Check sheet for the modelled part. Datum: model origin and axes. Units: mm. Face numbers are marked on the shaded views. A direction names the side the tool comes from. Round coordinates to 2 decimals unless told otherwise and drop trailing zeros. Write each loop counter-clockwise with the first axis right and the second up, starting at its lowest first coordinate (ties: lowest second). Pieces come first, ordered by that corner, then holes.
Item 1: Cross-section at A-A on y = 42. Enter the section's corners in (x, z), plus the area to 3 significant figures.
Item 2: Cross-section at D-D on x = 3. Enter the section's corners in (y, z).
Item 3: Material ranges on line 1 (Y direction, x = 7.25, z = 1.65); line 2 (Y direction, x = 31.75, z = 2.6); line 3 (X direction, y = 21.5, z = 6.25), recorded low to high.
Item 4: Cross-section at B-B on x = 15. Enter the section's corners in (y, z).
Item 5: Go/stop test with flat-tipped pins: pin 1 Ø3 at (x, y) = (31.75, 7.25) entering from -Z; pin 2 Ø6 at (y, z) = (26.5, -2) entering from -X; pin 3 Ø1 at (y, z) = (20, -1.5) entering from -X. Record where each tip stops, or that it passes through.
Item 6: Tool access check on the marked faces 1, 2 and 3. Record the directions out of +Z, -Z, +X, -X, +Y, -Y that give a thin tool (end or side, any length) a straight path to the whole face; none if there is none.
Item 7: Release check for a two-part mould opening along Y. For the marked faces 4, 5 and 6 record: +Y half, -Y half, draft (parallel to the pull), parting line (faces both ways), or undercut.
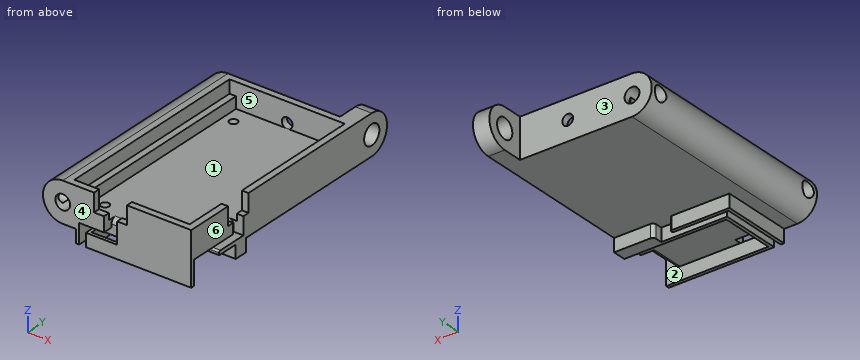
from build123d import *

# Parameters (mm, degrees)
SKETCH1_W                = 39
SKETCH1_H                = 65
BASE_DEPTH               = 4.5
SKETCH2_W                = 4
SKETCH2_H                = 57
WALLS_DEPTH              = 7.5
SKETCH3_W                = 10
SKETCH3_H                = 7.5
PWR_CONNECTOR_HOLE_DEPTH = 4
SKETCH4_W                = 7.5
SKETCH4_H                = 8
GPS_CONNECTOR_HOLE_DEPTH = 4
SKETCH5_R                = 1.25
MOUNTING_HOLES_DEPTH     = 4
GPS_MOUNT_DEPTH          = 4
SKETCH11_W               = 17
SKETCH11_H               = 1
SKETCH11_W_2             = 12
SKETCH11_H_2             = 3
PWR_CABLE_HOLDER1_DEPTH  = 4
SKETCH12_W               = 4
SKETCH12_H               = 2.5
PWR_CABLE_HOLDER2_DEPTH  = 3
PWR_FILLET_R             = 1.5
PWR_FILLET2_R            = 1
PWR_FILLET3_R            = 0.5
GPS_CABLE_HOLDER_DEPTH   = 3
GPS_START                = 1
GPS_FILLET_DEPTH         = 10
GPS_START_2              = 16.5
GPS_FILLET_2_DEPTH       = 4
GPS_START_3              = 9.15727
GPS_FILLET_3_DEPTH       = 8.34273
GPS_FILLET2_R            = 0.5
SKETCH15_R               = 6
BALLON_MOUNT_DEPTH       = 65
SKETCH16_R               = 2.25
BALLOON_MOUNT_HOLE_DEPTH = 65
SKETCH21_R               = 2.25
SAFETY_MOUNT_DEPTH       = 4.5
SKETCH22_W               = 35
SKETCH22_H               = 61
LID_HOLE_DEPTH           = 7.5
SKETCH25_W               = 3.5
SKETCH25_H               = 61
CORRECTION_DEPTH         = 2
SKETCH28_W               = 2
SKETCH28_H               = 2
SKETCH28_W_2             = 3
SMALL_WALLS_DEPTH        = 2
ANTENNA_MOUNTING_DEPTH   = 5
SKETCH30_R               = 3
ANTENNA_HOLE_DEPTH       = 5
SKETCH31_R               = 1.65
CABLE_HOLE_DEPTH         = 2


with BuildPart() as part:
    # Sketch1 → Base (new body)
    with BuildSketch(Plane.XY):
        with Locations((19.5, 32.5)):
            Rectangle(SKETCH1_W, SKETCH1_H)
    extrude(amount=BASE_DEPTH)

    # Sketch2 → Walls (add)
    with BuildSketch(Plane.XY.offset(4.5)):
        Polygon((39, 61), (39, 65), (0, 65), (0, 61), (4, 61), (35, 61), align=None)
        with Locations((37, 32.5)):
            Rectangle(SKETCH2_W, SKETCH2_H)
        Polygon((4, 61), (0, 61), (0, 0), (4, 0), (4, 4), align=None)
        Polygon((39, 0), (39, 4), (35, 4), (4, 4), (4, 0), align=None)
    extrude(amount=WALLS_DEPTH)

    # Sketch3 → PWR connector hole (cut)
    with BuildSketch(Plane(origin=(0, 4, 0), x_dir=(1, 0, 0), z_dir=(0, 1, 0))):
        with Locations((14.5, -8.25)):
            Rectangle(SKETCH3_W, SKETCH3_H)
    extrude(amount=-PWR_CONNECTOR_HOLE_DEPTH, mode=Mode.SUBTRACT)

    # Sketch4 → GPS connector hole (cut)
    with BuildSketch(Plane.ZY.offset(-35)):
        with Locations((8.25, 18.5)):
            Rectangle(SKETCH4_W, SKETCH4_H)
    extrude(amount=-GPS_CONNECTOR_HOLE_DEPTH, mode=Mode.SUBTRACT)

    # Sketch5 → Mounting holes (cut)
    with BuildSketch(Plane.XY.offset(4.5)):
        with Locations((7.25, 7.25)):
            Circle(SKETCH5_R)
        with Locations(Location((31.75, 7.25, 0), (0, 0, 180))):
            Circle(SKETCH5_R)
        with Locations(Location((7.25, 57.75, 0), (0, 0, 180))):
            Circle(SKETCH5_R)
        with Locations((31.75, 57.75)):
            Circle(SKETCH5_R)
    extrude(amount=-MOUNTING_HOLES_DEPTH, mode=Mode.SUBTRACT)

    # Sketch7 → GPS mount (add)
    with BuildSketch(Plane(origin=(0, 0, 0), x_dir=(-1, 0, 0), z_dir=(0, 0, -1))):
        Polygon((-39, 1), (-39, 0), (-7, 0), (-7, 18.5), (-39, 18.5), (-39, 17.5), (-8, 17.5), (-8, 1), align=None)
    extrude(amount=GPS_MOUNT_DEPTH)

    # Sketch11 → PWR cable holder1 (add)
    with BuildSketch(Plane(origin=(0, 0, 0), x_dir=(-1, 0, 0), z_dir=(0, 0, -1))):
        Polygon((-5, 0), (-4, 0), (-4, 21.5), (-5, 21.5), (-5, 20.5), align=None)
        with Locations((-13.5, 21)):
            Rectangle(SKETCH11_W, SKETCH11_H)
        with Locations((-33, 20)):
            Rectangle(SKETCH11_W_2, SKETCH11_H_2)
    extrude(amount=PWR_CABLE_HOLDER1_DEPTH)

    # Sketch12 → PWR cable holder2 (cut)
    with BuildSketch(Plane.XZ):
        Polygon((5, 2), (5, 0), (7, 0), (16.5, 0), (16.5, 2), (12.5, 2), align=None)
        with Locations((14.5, 3.25)):
            Rectangle(SKETCH12_W, SKETCH12_H)
    extrude(amount=-PWR_CABLE_HOLDER2_DEPTH, mode=Mode.SUBTRACT)

    # PWR fillet
    pwr_fillet_edges = [part.edges().sort_by_distance(p)[0] for p in [
        (6, 3, 0),
        (14.5, 3, 4.5),
    ]]
    fillet(pwr_fillet_edges, radius=PWR_FILLET_R)

    # PWR fillet2
    pwr_fillet2_edges = [part.edges().sort_by_distance(p)[0] for p in [
        (27, 21.5, -2),
    ]]
    fillet(pwr_fillet2_edges, radius=PWR_FILLET2_R)

    # PWR fillet3
    pwr_fillet3_edges = [part.edges().sort_by_distance(p)[0] for p in [
        (22, 21.5, -2),
        (22, 20.5, -2),
    ]]
    fillet(pwr_fillet3_edges, radius=PWR_FILLET3_R - 0.0001)  # a hair under: the kernel refuses the full size

    # Sketch13 → GPS cable holder (cut)
    with BuildSketch(Plane(origin=(39, 0, 0), x_dir=(0, 0, -1), z_dir=(1, 0, 0))):
        Polygon((-1.156586719, 11), (-2.326586719, 11), (-2.326586719, 1), (0, 1), (0, 11), align=None)
        Polygon((-2.326586719, 11), (-2.326586719, 16.5), (-3.326586719, 16.5), (-3.326586719, 1), (-2.326586719, 1), align=None)
        Polygon((-1.156586719, 20.5), (-2.326586719, 20.5), (-2.326586719, 16.5), (-2.326586719, 11), (-1.156586719, 11), align=None)
        Polygon((-2.326586719, 20.5), (-4.5, 20.5), (-4.5, 16.5), (-3.326586719, 16.5), (-2.326586719, 16.5), align=None)
    extrude(amount=-GPS_CABLE_HOLDER_DEPTH, mode=Mode.SUBTRACT)

    # GPS fillet: read off the stored shape, not the designer's step
    # GPS fillet outline → GPS fillet (cut)
    with BuildSketch(Plane(origin=(0, 0, 0), x_dir=(1, 0, 0), z_dir=(0, 1, 0)).offset(GPS_START)):
        with BuildLine():
            Line((36, -3.326586719), (36, -3.25))
            ThreePointArc((36, -3.25), (35.999412758, -3.288311358), (35.997651584, -3.326586719))
            Line((35.997651584, -3.326586719), (36, -3.326586719))
        make_face()
        with BuildLine():
            Line((36, -1.25), (36, 0))
            Line((36, 0), (34.75, 0))
            ThreePointArc((34.75, 0), (35.633883476, -0.366116524), (36, -1.25))
        make_face()
    extrude(amount=GPS_FILLET_DEPTH, mode=Mode.SUBTRACT)

    # GPS fillet 2 outline → GPS fillet 2 (cut)
    with BuildSketch(Plane(origin=(0, 0, 0), x_dir=(1, 0, 0), z_dir=(0, 1, 0)).offset(GPS_START_2)):
        with BuildLine():
            ThreePointArc((36, -3.25), (35.633883476, -4.133883476), (34.75, -4.5))
            Line((34.75, -4.5), (36, -4.5))
            Line((36, -4.5), (36, -3.25))
        make_face()
        with BuildLine():
            ThreePointArc((35.996504697, -1.156586719), (35.999125868, -1.203260674), (36, -1.25))
            Line((36, -1.25), (36, -1.156586719))
            Line((36, -1.156586719), (35.996504697, -1.156586719))
        make_face()
    extrude(amount=GPS_FILLET_2_DEPTH, mode=Mode.SUBTRACT)

    # GPS fillet 3 outline → GPS fillet 3 (cut)
    with BuildSketch(Plane(origin=(0, 0, 0), x_dir=(1, 0, 0), z_dir=(0, 1, 0)).offset(GPS_START_3)):
        with BuildLine():
            Line((36, -3.326586719), (36, -3.25))
            ThreePointArc((36, -3.25), (35.999412758, -3.288311358), (35.997651584, -3.326586719))
            Line((35.997651584, -3.326586719), (36, -3.326586719))
        make_face()
        with BuildLine():
            ThreePointArc((35.996504697, -1.156586719), (35.999125868, -1.203260674), (36, -1.25))
            Line((36, -1.25), (36, -1.156586719))
            Line((36, -1.156586719), (35.996504697, -1.156586719))
        make_face()
    extrude(amount=GPS_FILLET_3_DEPTH, mode=Mode.SUBTRACT)

    # GPS fillet2
    # the kernel refuses this fillet: 0.5 mm, written as the material it takes off along each edge
    with BuildSketch(Plane(origin=(40.25, 11, 1.156586719), x_dir=(0, 0, -1), z_dir=(-1, 0, 0))) as gps_fillet2_piece_1:
        with BuildLine():
            CenterArc((GPS_FILLET2_R, -GPS_FILLET2_R), GPS_FILLET2_R, 90, 90)
            Line((0, -GPS_FILLET2_R), (0, 0))
            Line((0, 0), (GPS_FILLET2_R, 0))
        make_face()
    extrude(amount=4.25, mode=Mode.SUBTRACT)
    with BuildSketch(Plane(origin=(40.25, 16.5, 3.326586719), x_dir=(0, -1, 0), z_dir=(-1, 0, 0))) as gps_fillet2_piece_2:
        with BuildLine():
            CenterArc((GPS_FILLET2_R, GPS_FILLET2_R), GPS_FILLET2_R, 180, 90)
            Line((0, GPS_FILLET2_R), (0, 0))
            Line((0, 0), (GPS_FILLET2_R, 0))
        make_face()
    extrude(amount=4.25, mode=Mode.SUBTRACT)
    with BuildSketch(Plane(origin=(36, 16.5, 3.326586719), x_dir=(0, -1.0, 5.126796764898245e-10), z_dir=(-1, 0, 0))) as gps_fillet2_piece_3_section:
        with BuildLine():
            CenterArc((GPS_FILLET2_R, GPS_FILLET2_R), GPS_FILLET2_R, 179.999999971, 90)
            Line((GPS_FILLET2_R * 5.12679676753e-10, GPS_FILLET2_R), (0, 0))
            Line((0, 0), (GPS_FILLET2_R, 0))
        make_face()
    gps_fillet2_piece_3 = extrude(amount=1.252348417, mode=Mode.PRIVATE)
    gps_fillet2_piece_3 = gps_fillet2_piece_3 - Plane(origin=(34.749999755, 16.5, 3.249999996), x_dir=(1.0, 0, 2.949740140725451e-09), z_dir=(0, -1, 0)) * Cylinder(1.250000245, 5, mode=Mode.PRIVATE)
    add(gps_fillet2_piece_3, mode=Mode.SUBTRACT)
    with BuildSketch(Plane(origin=(34.746504697, 11, 1.156586719), x_dir=(0, 0, -1), z_dir=(1, 0, 0))) as gps_fillet2_piece_4_section:
        with BuildLine():
            CenterArc((GPS_FILLET2_R, GPS_FILLET2_R), GPS_FILLET2_R, 180, 90)
            Line((-GPS_FILLET2_R * 5.12674791509e-10, GPS_FILLET2_R), (0, 0))
            Line((0, 0), (GPS_FILLET2_R, 0))
        make_face()
    gps_fillet2_piece_4 = extrude(amount=1.253495303, mode=Mode.PRIVATE)
    gps_fillet2_piece_4 = gps_fillet2_piece_4 - Plane(origin=(34.749999998, 11, 1.250000002), x_dir=(1.3197563913171698e-09, 0, -1.0), z_dir=(0, -1, 0)) * Cylinder(1.250000002, 5, mode=Mode.PRIVATE)
    add(gps_fillet2_piece_4, mode=Mode.SUBTRACT)

    # Sketch15 → Ballon mount (add)
    with BuildSketch(Plane.XZ):
        with Locations((0, 6)):
            Circle(SKETCH15_R)
    extrude(amount=-BALLON_MOUNT_DEPTH)

    # Sketch16 → Balloon mount hole (cut)
    with BuildSketch(Plane.XZ):
        with Locations(Location((0, 6, 0), (0, 0, 270))):
            Circle(SKETCH16_R)
    extrude(amount=-BALLOON_MOUNT_HOLE_DEPTH, mode=Mode.SUBTRACT)

    # Sketch21 → Safety mount (cut)
    with BuildSketch(Plane.ZY.offset(6)):
        with Locations((6, 3.5)):
            Circle(SKETCH21_R)
        with Locations((6, 61.5)):
            Circle(SKETCH21_R)
    extrude(amount=-SAFETY_MOUNT_DEPTH, mode=Mode.SUBTRACT)

    # Sketch22 → Lid hole (cut)
    with BuildSketch(Plane.XY.offset(12)):
        with Locations((19.5, 32.5)):
            Rectangle(SKETCH22_W, SKETCH22_H)
    extrude(amount=-LID_HOLE_DEPTH, mode=Mode.SUBTRACT)

    # Sketch25 → Correction (add)
    with BuildSketch(Plane(origin=(2, 0, 0), x_dir=(0, 0, -1), z_dir=(1, 0, 0))):
        with Locations((-6.25, 32.5)):
            Rectangle(SKETCH25_W, SKETCH25_H)
    extrude(amount=CORRECTION_DEPTH)

    # Sketch28 → Small walls (add)
    with BuildSketch(Plane.XY.offset(4.5)):
        with Locations((38, 21.5)):
            Rectangle(SKETCH28_W, SKETCH28_H)
        with Locations((38, 15.5)):
            Rectangle(SKETCH28_W, SKETCH28_H)
        with Locations((18, 1)):
            Rectangle(SKETCH28_W_2, SKETCH28_H)
        with Locations((11, 1)):
            Rectangle(SKETCH28_W_2, SKETCH28_H)
    extrude(amount=SMALL_WALLS_DEPTH)

    # Sketch29 → Antenna mounting (add)
    with BuildSketch(Plane(origin=(39, 0, 0), x_dir=(0, 0, -1), z_dir=(1, 0, 0))):
        with BuildLine():
            Line((0, 65), (0, 71))
            ThreePointArc((0, 71), (-6, 77), (-12, 71))
            Line((-12, 71), (-12, 65))
            Line((-12, 65), (0, 65))
        make_face()
    extrude(amount=-ANTENNA_MOUNTING_DEPTH)

    # Sketch30 → Antenna hole (cut)
    with BuildSketch(Plane(origin=(39, 0, 0), x_dir=(0, 0, -1), z_dir=(1, 0, 0))):
        with Locations((-6, 71)):
            Circle(SKETCH30_R)
    extrude(amount=-ANTENNA_HOLE_DEPTH, mode=Mode.SUBTRACT)

    # Sketch31 → Cable hole (cut)
    with BuildSketch(Plane(origin=(0, 65, 0), x_dir=(1, 0, 0), z_dir=(0, 1, 0))):
        with Locations(Location((19.5, -6, 0), (0, 0, 270))):
            Circle(SKETCH31_R)
    extrude(amount=-CABLE_HOLE_DEPTH, mode=Mode.SUBTRACT)


solid = part.part
Response values:
1. outline: (0, 0) - (39, 0) - (39, 12) - (37, 12) - (37, 4.5) - (4, 4.5) - (4, 8) - (2, 8) - (2, 12) - (0, 12) arc R6 ccw to start; hole (2, 4.97) - (2, 7.03) arc R2.25 ccw (long way) to start
1. area: 253 mm2
2. outline: (0, 0) - (65, 0) - (65, 12) - (63, 12) - (63, 8) - (2, 8) - (2, 12) - (0, 12) - close
3. line 1: y = 3 to 6, 8.5 to 56.5, 59 to 65
3. line 2: y = 0 to 6, 8.5 to 56.5, 59 to 65
3. line 3: x = -5.99 to -2.24, 2 to 4, 37 to 39
4. outline: (0, -4) - (1, -4) - (1, 0) - (0, 0) - close; (3, 0) - (17.5, 0) - (17.5, -4) - (18.5, -4) - (18.5, 0) - (20.5, 0) - (20.5, -4) - (21.5, -4) - (21.5, 0) - (65, 0) - (65, 12) - (63, 12) - (63, 4.5) - (4.5, 4.5) arc R1.5 ccw to (3, 3) - close
5. pin 1: stops at z = 0
5. pin 2: stops at x = -3.32
5. pin 3: stops at x = 4
6. face 1: +Z
6. face 2: -Z, +X
6. face 3: +Z, -Z, -X, +Y
7. face 4: -Y half
7. face 5: undercut
7. face 6: draft
